Geometry: final body of the model. Coordinates: model frame, mm. A direction names the side the tool comes from. Coordinates: 2 decimals unless noted, no trailing zeros. Loops run counter-clockwise (first coordinate to the right, second up) from the corner with the lowest first, then second, coordinate; pieces in that order, holes last. Notation, with made-up numbers: (13.25, 0.25) - (71.25, 0.25) arc R22 cw to (71.25, 15.25) - close; hole circle Ø9 at (-36, 16.25). An arc over 180 degrees is marked (long way). Answer in a Markdown table with one row per item.
from build123d import *

# Parameters (mm, degrees)
F0_W         = 44
F0_H         = 44
F1_DEPTH     = 70
F2_W         = 40
F2_H         = 42
F3_DEPTH     = 70
F5_DEPTH     = 44
F7_DEPTH     = 2
F9_W         = 8
F9_H         = 8
F10_DEPTH    = 80
F11_W        = 8
F11_H        = 2
F12_DEPTH    = 12
F13_W        = 20
F13_H        = 8
F14_DEPTH    = 50
F15_W        = 15
F15_H        = 2
F16_DEPTH    = 50
F17_R        = 3.9
F18_DEPTH    = 20
F19_SIZE2    = 1.5
F19_SIZE     = 7
F20_SIZE2    = 7
F20_SIZE     = 1.5
F21_SIZE2    = 7
F21_SIZE     = 1.5
F22_R        = 1.75
F23_DEPTH    = 8
F24_DEPTH    = 44
F25_W        = 8
F25_H        = 8
F25_R        = 0.75
F26_DEPTH    = 8
F27_R        = 1.75
F28_DEPTH    = 8
F29_T1_DEPTH = 28
F30_W        = 8
F30_H        = 8
F30_R        = 0.75
F31_DEPTH    = 8
F32_R        = 1.75
F33_DEPTH    = 8
F34_T1_DEPTH = 28


# Not quite as in the source:
# - a fillet or chamfer that OpenCascade refuses, or shapes differently, is made with other operations: its cross-section is extruded or revolved along the edge and cut away or added


with BuildPart() as f1:
    # F0 (on Front) → F1 (new body)
    with BuildSketch(Plane.XZ):
        with Locations((22, 22)):
            Rectangle(F0_W, F0_H)
    extrude(amount=-F1_DEPTH)

    # F2 (on face) → F3 (cut, through all)
    with BuildSketch(Plane.XZ):
        with Locations((22, 21)):
            Rectangle(F2_W, F2_H)
    extrude(amount=-F3_DEPTH, mode=Mode.SUBTRACT)

    # F4 (on face) → F5 (cut)
    with BuildSketch(Plane.YZ.offset(44)):
        with BuildLine():
            ThreePointArc((51.25, 37.25), (49, 39.5), (46.75, 37.25))
            Line((46.75, 37.25), (46.75, 17.25))
            ThreePointArc((46.75, 17.25), (49, 15), (51.25, 17.25))
            Line((51.25, 17.25), (51.25, 37.25))
        make_face()
    extrude(amount=-F5_DEPTH, mode=Mode.SUBTRACT)

    # F6 (on face) → F7 (cut, through all)
    with BuildSketch(Plane.XY.offset(44)):
        with BuildLine():
            Line((2, 51), (2, 0))
            Line((2, 0), (42, 0))
            Line((42, 0), (42, 51))
            ThreePointArc((42, 51), (40.5355339059, 54.5355339059), (37, 56))
            Line((37, 56), (7, 56))
            ThreePointArc((7, 56), (3.4644660941, 54.5355339059), (2, 51))
        make_face()
    extrude(amount=-F7_DEPTH, mode=Mode.SUBTRACT)

    # F9 (on face) → F10 (join)
    with BuildSketch(Plane.YZ.offset(44)):
        with Locations((35, 8)):
            Rectangle(F9_W, F9_H)
    extrude(amount=F10_DEPTH)

    # F11 (on face) → F12 (cut)
    with BuildSketch(Plane.YZ.offset(124)):
        with Locations((35, 11)):
            Rectangle(F11_W, F11_H)
    extrude(amount=-F12_DEPTH, mode=Mode.SUBTRACT)

    # F13 (on face) → F14 (join)
    with BuildSketch(Plane(origin=(0, 0, 0), x_dir=(0, -1, 0), z_dir=(-1, 0, 0))):
        with Locations((-23.5, 19)):
            Rectangle(F13_W, F13_H)
    extrude(amount=F14_DEPTH)

    # F15 (on face) → F16 (cut, through all)
    with BuildSketch(Plane(origin=(-50, 0, 0), x_dir=(0, -1, 0), z_dir=(-1, 0, 0))):
        with Locations((-23.5, 16)):
            Rectangle(F15_W, F15_H)
    extrude(amount=-F16_DEPTH, mode=Mode.SUBTRACT)

    # F17 (on face) → F18 (cut)
    with BuildSketch(Plane.XY.offset(23)):
        with Locations((-35, 23.5)):
            Circle(F17_R)
    extrude(amount=-F18_DEPTH, mode=Mode.SUBTRACT)

    # F19
    f19_edges = [f1.edges().sort_by_distance(p)[0] for p in [
        (44, 70, 22),
    ]]
    f19_side = f1.faces().sort_by_distance((44, 34.490511, 22.116835))[0]
    chamfer(f19_edges, length=F19_SIZE, length2=F19_SIZE2, reference=f19_side)

    # F20
    f20_edges = [f1.edges().sort_by_distance(p)[0] for p in [
        (21.25, 70, 44),
    ]]
    f20_side = f1.faces().sort_by_distance((21.25, 70, 43.388261))[0]
    chamfer(f20_edges, length=F20_SIZE, length2=F20_SIZE2, reference=f20_side)

    # F21
    f21_edges = [f1.edges().sort_by_distance(p)[0] for p in [
        (0, 70, 21.25),
    ]]
    f21_side = f1.faces().sort_by_distance((42.439896, 70, 21.25))[0]
    chamfer(f21_edges, length=F21_SIZE, length2=F21_SIZE2, reference=f21_side)

    # F22 (on face) → F23 (cut)
    with BuildSketch(Plane.XY.offset(10)):
        with Locations((118, 35)):
            Circle(F22_R)
    extrude(amount=-F23_DEPTH, mode=Mode.SUBTRACT)

    # F8 (on face) → F24 (cut)
    with BuildSketch(Plane.YZ.offset(44)):
        with BuildLine():
            ThreePointArc((10.25, 37.25), (8, 39.5), (5.75, 37.25))
            Line((5.75, 37.25), (5.75, 17.25))
            ThreePointArc((5.75, 17.25), (8, 15), (10.25, 17.25))
            Line((10.25, 17.25), (10.25, 37.25))
        make_face()
    extrude(amount=-F24_DEPTH, mode=Mode.SUBTRACT)

    # F25 (on face) → F26 (join)
    with BuildSketch(Plane.YZ.offset(44)):
        with Locations((58, 13)):
            Rectangle(F25_W, F25_H)
        with Locations((58, 13)):
            Circle(F25_R, mode=Mode.SUBTRACT)
    extrude(amount=F26_DEPTH)

    # F27 (on face) → F28 (cut)
    with BuildSketch(Plane.XY.offset(17)):
        with Locations((48, 58)):
            Circle(F27_R)
    extrude(amount=-F28_DEPTH, mode=Mode.SUBTRACT)

    # F29: fillet of radius 4 on 1 edges, made by hand

    # F29_s2 → F29_t1 (cut)
    with BuildSketch(Plane.XY.offset(-1)):
        with BuildLine():
            ThreePointArc((48, 62), (50.8284271247, 60.8284271247), (52, 58))
            Line((52, 58), (52, 62))
            Line((52, 62), (48, 62))
        make_face()
    extrude(amount=F29_T1_DEPTH, mode=Mode.SUBTRACT)

    # F30 (on face) → F31 (join)
    with BuildSketch(Plane(origin=(0, 0, 0), x_dir=(0, -1, 0), z_dir=(-1, 0, 0))):
        with Locations((-58, 13)):
            Rectangle(F30_W, F30_H)
        with Locations((-58, 13)):
            Circle(F30_R, mode=Mode.SUBTRACT)
    extrude(amount=F31_DEPTH)

    # F32 (on face) → F33 (cut)
    with BuildSketch(Plane.XY.offset(17)):
        with Locations((-4, 58)):
            Circle(F32_R)
    extrude(amount=-F33_DEPTH, mode=Mode.SUBTRACT)

    # F34: fillet of radius 4 on 1 edges, made by hand

    # F34_s2 → F34_t1 (cut)
    with BuildSketch(Plane.XY.offset(-1)):
        with BuildLine():
            ThreePointArc((-4, 62), (-6.8284271247, 60.8284271247), (-8, 58))
            Line((-8, 58), (-8, 62))
            Line((-8, 62), (-4, 62))
        make_face()
    extrude(amount=F34_T1_DEPTH, mode=Mode.SUBTRACT)


solid = f1.part
(1) First-contact query: pin 1 Ø2 at (x, y) = (48, 58) entering from +Z; pin 2 Ø1.2 at (y, z) = (58, 13) entering from +X; pin 3 Ø0.6 at (x, z) = (-27.5, 15.5) entering from +Y; pin 4 Ø1.2 at (y, z) = (56, 12) entering from +X. Flat tips, straight axial feed; report the tip coordinate or a pass-through.
Verdict:
| item | result |
|---|---|
| pin 1 | passes through |
| pin 2 | stops at x = 44 |
| pin 3 | stops at y = 33.5 |
| pin 4 | stops at x = 52 |
(2) Pull-direction query (Y, two-part tool) for faces 6 (the face through (48, 56, 17)), 7 (the face through (21.69, 66.45, 43.26)), 8 (the face through (119.669, 35.526, 7.042)); classes: pulls with the +Y half, pulls with the -Y half, needs draft (parallel to the pull), parting line crosses it, or undercut.
Verdict:
| item | result |
|---|---|
| face 6 | needs draft |
| face 7 | pulls with the +Y half |
| face 8 | undercut |
(3) Cut plane C-C on y = 23.5. Output: boundary loops of the cut face in (x, z), then the cut area to 3 significant figures.
Verdict:
| item | result |
|---|---|
| outline | (-50, 17) - (-38.9, 17) - (-38.9, 23) - (-50, 23) - close; (-31.1, 17) - (0, 17) - (0, 0) - (2, 0) - (2, 44) - (0, 44) - (0, 23) - (-31.1, 23) - close; (42, 0) - (44, 0) - (44, 44) - (42, 44) - close |
| area | 429 mm² |
(4) Cut plane B-B on x = -35. Output: boundary loops of the cut face in (y, z).
Verdict:
| item | result |
|---|---|
| outline | (13.5, 15) - (16, 15) - (16, 17) - (19.6, 17) - (19.6, 23) - (13.5, 23) - close; (27.4, 17) - (31, 17) - (31, 15) - (33.5, 15) - (33.5, 23) - (27.4, 23) - close |
(5) Cut plane A-A on z = 28. Output: boundary loops of the cut face in (x, y).
Verdict:
| item | result |
|---|---|
| outline | (0, 0) - (2, 0) - (2, 5.75) - (0, 5.75) - close; (0, 10.25) - (2, 10.25) - (2, 46.75) - (0, 46.75) - close; (0, 51.25) - (2, 51.25) - (2, 70) - (1.5, 70) - (0, 63) - close; (42, 0) - (44, 0) - (44, 5.75) - (42, 5.75) - close; (42, 10.25) - (44, 10.25) - (44, 46.75) - (42, 46.75) - close; (42, 51.25) - (44, 51.25) - (44, 63) - (42.5, 70) - (42, 70) - close |
(6) Cut plane D-D on y = 49. Output: boundary loops of the cut face in (x, z).
Verdict:
| item | result |
|---|---|
| outline | (0, 0) - (2, 0) - (2, 15) - (0, 15) - close; (0, 39.5) - (2, 39.5) - (2, 44) - (0, 44) - close; (42, 0) - (44, 0) - (44, 15) - (42, 15) - close; (42, 39.5) - (44, 39.5) - (44, 44) - (42, 44) - close |
(7) Access query for faces 1 (the face through (22, 62, 42)), 2 (the face through (-2, 58, 9)), 3 (the face through (-25, 24, 23)), 4 (the face through (-2, 58, 17)), 5 (the face through (83, 31, 8)). Directions: +Z, -Z, +X, -X, +Y, -Y. A direction counts if a zero-diameter tool reaches every point of the face in a straight line with its end or side. Return the directions, or none.
Verdict:
| item | result |
|---|---|
| face 1 | -Z, +Y, -Y |
| face 2 | -Z, -X, +Y, -Y |
| face 3 | +Z, -X, +Y, -Y |
| face 4 | +Z, -X, +Y |
| face 5 | +Z, -Z, +X, -Y |
(8) Ray query, probe 1 along Y at (x, z) = (48, 11); probe 2 along X at (y, z) = (39.5, 39.5); probe 3 along Y at (x, z) = (-35, 20.65). Return the intervals inside material, ascending.
Verdict:
| item | result |
|---|---|
| probe 1 | y = 31 to 39, 54 to 56.25, 59.75 to 62 |
| probe 2 | x = 0 to 2, 42 to 44 |
| probe 3 | y = 13.5 to 19.6, 27.4 to 33.5 |
